Geometry: see drawing. Coordinates: mm, zero at the bounding-box minimum. A direction names the side the tool comes from. Coordinates: 2 decimals unless noted, no trailing zeros. Loops run counter-clockwise (first coordinate to the right, second up) from the corner with the lowest first, then second, coordinate; pieces in that order, holes last. Notation, with made-up numbers: (-8.75, 47.5) -> (8.25, 47.5) arc R27 ccw to (8.25, 77.5) -> close; hole circle Ø3 at (70, 50). An arc over 180 degrees is marked (long way). One line per item, written item: value. Start each with the question number.
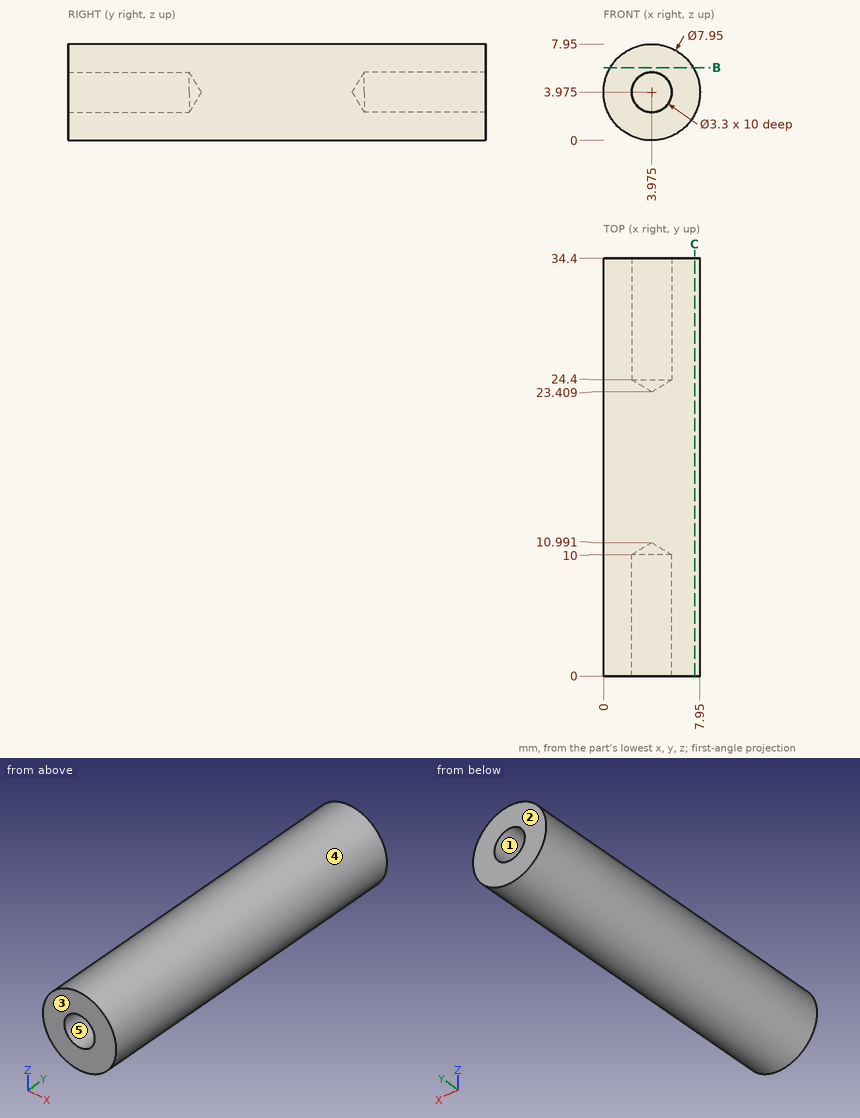
1. Section B-B on z = 6. Return the cut outline in (x, y) (1 decimal), plus the area to 3 significant figures.
2. Pin query (flat end, axial travel): pin 1 Ø1 at (y, z) = (16, 5.5) entering from +X; pin 2 Ø2 at (x, z) = (3.98, 3.98) entering from -Y. Return the tip coordinate at first contact, or that it passes through.
3. Set-up query: the marked faces 1 and 2. Return all of +Z, -Z, +X, -X, +Y, -Y with unobstructed straight access to the full face (end or side cutting, diameter ignored); none if empty.
4. Draft query along Z for the marked faces 3, 4 and 5. Return one class per face: released by +Z, released by -Z, zero draft, split by the parting line, or undercut.
5. Section C-C on x = 7.5. Return the cut outline in (y, z), plus the area to 3 significant figures.
6. Line query: L1, parallel to Z at x = 5.25, y = 28 (1 decimal); L2, parallel to X at y = 26.5, z = 3 (1 decimal); L3, parallel to Z at x = 3.25, y = 9.5 (1 decimal). Output: solid intervals per line, ascending. Write a range as [from, to].
Checks:
1. outline: (0.6, 0) -> (7.4, 0) -> (7.4, 34.4) -> (0.6, 34.4) -> close
1. area: 235 mm²
2. pin 1: x = 7.82
2. pin 2: y = 10.39
3. face 1: +Y
3. face 2: +Z, -Z, +X, -X, +Y
4. face 3: zero draft
4. face 4: split by the parting line
4. face 5: undercut
5. outline: (0, 2.14) -> (34.4, 2.14) -> (34.4, 5.81) -> (0, 5.81) -> close
5. area: 126 mm²
6. L1: [0.2, 2.9], [5, 7.7]
6. L2: [0.1, 2.6], [5.3, 7.8]
6. L3: [0.1, 2.5], [5.5, 7.9]
